from build123d import *

# Parameters (mm, degrees)
BASE_FLANGE1_DEPTH      = 25.4
BASE_FLANGE2_DEPTH      = 7.62
BASE_FLANGE2_DEPTH_BACK = 7.62
SKETCH9_R               = 2.159
CUT_EXTRUDE1_DEPTH      = 1.6764
SKETCH12_R              = 1.6764
SKETCH12_R_2            = 2.159
CUT_EXTRUDE4_DEPTH      = 1.6764
CUT_EXTRUDE5_DEPTH      = 2.54


# Sheet-metal steps are written as plain solids
with BuildPart() as part:
    # Sketch1 → Base-Flange1 (new body)
    with BuildSketch(Plane.XY):
        with BuildLine():
            Line((-52.705, -15.875), (-52.705, 15.3924))
            ThreePointArc((-52.705, 15.3924), (-52.563649733, 15.733649733), (-52.2224, 15.875))
            Line((-52.2224, 15.875), (52.2224, 15.875))
            ThreePointArc((52.2224, 15.875), (52.563649733, 15.733649733), (52.705, 15.3924))
            Line((52.705, 15.3924), (52.705, -15.875))
            Line((52.705, -15.875), (54.3814, -15.875))
            Line((54.3814, -15.875), (54.3814, 15.3924))
            ThreePointArc((54.3814, 15.3924), (53.749043541, 16.919043541), (52.2224, 17.5514))
            Line((52.2224, 17.5514), (-52.2224, 17.5514))
            ThreePointArc((-52.2224, 17.5514), (-53.749043541, 16.919043541), (-54.3814, 15.3924))
            Line((-54.3814, 15.3924), (-54.3814, -15.875))
            Line((-54.3814, -15.875), (-52.705, -15.875))
        make_face()
    extrude(amount=BASE_FLANGE1_DEPTH)


with BuildPart() as body_2:
    # Sketch6 → Base-Flange2 (new, two sides: drawn at the far end of the back side and taken through both)
    with BuildSketch(Plane(origin=(0, 0, 0), x_dir=(0, 0, -1), z_dir=(1, 0, 0)).offset(-BASE_FLANGE2_DEPTH_BACK)):
        with BuildLine():
            Line((-25.4, 15.875), (-68.0974, 15.875))
            ThreePointArc((-68.0974, 15.875), (-68.438649733, 15.733649733), (-68.58, 15.3924))
            Line((-68.58, 15.3924), (-68.58, 5.334))
            ThreePointArc((-68.58, 5.334), (-69.212356459, 3.807356459), (-70.739, 3.175))
            Line((-70.739, 3.175), (-99.06, 3.175))
            Line((-99.06, 3.175), (-99.06, 4.8514))
            Line((-99.06, 4.8514), (-70.739, 4.8514))
            ThreePointArc((-70.739, 4.8514), (-70.397750267, 4.992750267), (-70.2564, 5.334))
            Line((-70.2564, 5.334), (-70.2564, 15.3924))
            ThreePointArc((-70.2564, 15.3924), (-69.624043541, 16.919043541), (-68.0974, 17.5514))
            Line((-68.0974, 17.5514), (-25.4, 17.5514))
            Line((-25.4, 17.5514), (-25.4, 15.875))
        make_face()
    extrude(amount=BASE_FLANGE2_DEPTH + BASE_FLANGE2_DEPTH_BACK)

    # Sketch9 → Cut-Extrude1 (cut)
    with BuildSketch(Plane(origin=(0, 4.8514, 0), x_dir=(1, 0, 0), z_dir=(0, 1, 0))):
        with Locations(Location((0, -78.3844, 0), (0, 0, 270))):
            Circle(SKETCH9_R)
        with Locations(Location((0, -93.4466, 0), (0, 0, 270))):
            Circle(SKETCH9_R)
    extrude(amount=-CUT_EXTRUDE1_DEPTH, mode=Mode.SUBTRACT)


with BuildPart() as cut_extrude4_tool:
    # Sketch12 → Cut-Extrude4 (new body)
    with BuildSketch(Plane(origin=(0, 17.5514, 0), x_dir=(1, 0, 0), z_dir=(0, 1, 0))):
        with Locations(Location((0, -57.15, 0), (0, 0, 270))):
            Circle(SKETCH12_R)
        with Locations(Location((-41.49725, -12.7, 0), (0, 0, 270))):
            Circle(SKETCH12_R_2)
        with Locations(Location((41.49725, -12.7, 0), (0, 0, 270))):
            Circle(SKETCH12_R_2)
    extrude(amount=-CUT_EXTRUDE4_DEPTH)


with BuildPart() as part_1:
    add(part.part)

    # Cut-Extrude4: cut by cut_extrude4_tool
    add(cut_extrude4_tool.part, mode=Mode.SUBTRACT)


with BuildPart() as body_2_1:
    add(body_2.part)

    # Cut-Extrude4: cut by cut_extrude4_tool
    add(cut_extrude4_tool.part, mode=Mode.SUBTRACT)


with BuildPart() as cut_extrude5_tool:
    # Sketch12<3> → Cut-Extrude5 (new body)
    with BuildSketch(Plane(origin=(0, 17.5514, 0), x_dir=(1, 0, 0), z_dir=(0, 1, 0))):
        with BuildLine():
            Line((-1.6764, -25.4), (1.6764, -25.4))
            ThreePointArc((1.6764, -25.4), (0, -23.7236), (-1.6764, -25.4))
        make_face()
        with BuildLine():
            ThreePointArc((-1.6764, -25.4), (0, -27.0764), (1.6764, -25.4))
            Line((1.6764, -25.4), (-1.6764, -25.4))
        make_face()
    extrude(amount=-CUT_EXTRUDE5_DEPTH)


with BuildPart() as part_2:
    add(part_1.part)

    # Cut-Extrude5: cut by cut_extrude5_tool
    add(cut_extrude5_tool.part, mode=Mode.SUBTRACT)


with BuildPart() as body_2_2:
    add(body_2_1.part)

    # Cut-Extrude5: cut by cut_extrude5_tool
    add(cut_extrude5_tool.part, mode=Mode.SUBTRACT)

    # Combine1: union part
    add(part_2.part)


solid = body_2_2.part
Check sheet for the modelled part. Datum: model origin and axes. Units: mm. A direction names the side the tool comes from. Coordinates: 2 decimals unless noted, no trailing zeros. Write each loop counter-clockwise with the first axis right and the second up, starting at its lowest first coordinate (ties: lowest second). Pieces come first, ordered by that corner, then holes.
Item 1: Mould release check, pull along X, two halves, no side actions. Record for faces 1 (the face through (0, 3.175, 85)), 2 (the face through (7.62, 16.3, 62.1)), 3 (the face through (-52.705, 0, 13)), 4 (the face through (-42.811, 16.725, 10.987)): released by +X, released by -X, zero draft, split by the parting line, or undercut.
Numbers:
face 1: zero draft
face 2: released by +X
face 3: undercut
face 4: undercut
Item 2: Cross-section at D-D on y = -10. Record the boundary of the cut face in (x, z) (3 decimals).
Numbers:
outline: (-54.381, 0) - (-52.705, 0) - (-52.705, 25.4) - (-54.381, 25.4) - close; (52.705, 0) - (54.381, 0) - (54.381, 25.4) - (52.705, 25.4) - close
Item 3: Cross-section at A-A on y = 14. Record the boundary of the cut face in (x, z) (3 decimals).
Numbers:
outline: (-54.381, 0) - (-52.705, 0) - (-52.705, 25.4) - (-54.381, 25.4) - close; (-7.62, 68.58) - (7.62, 68.58) - (7.62, 70.256) - (-7.62, 70.256) - close; (52.705, 0) - (54.381, 0) - (54.381, 25.4) - (52.705, 25.4) - close
Item 4: Cross-section at C-C on x = 0. Record the boundary of the cut face in (y, z) (3 decimals), then the cut area to 3 significant figures.
Numbers:
outline: (3.175, 70.739) arc R2.159 ccw to (5.334, 68.58) - (15.392, 68.58) arc R0.483 cw to (15.875, 68.097) - (15.875, 58.826) - (17.551, 58.826) - (17.551, 68.097) arc R2.159 ccw to (15.392, 70.256) - (5.334, 70.256) arc R0.483 cw to (4.851, 70.739) - (4.851, 76.225) - (3.175, 76.225) - close; (3.175, 80.543) - (4.851, 80.543) - (4.851, 91.288) - (3.175, 91.288) - close; (3.175, 95.606) - (4.851, 95.606) - (4.851, 99.06) - (3.175, 99.06) - close; (15.875, 0) - (17.551, 0) - (17.551, 23.724) - (15.875, 23.724) - close; (15.875, 27.076) - (17.551, 27.076) - (17.551, 55.474) - (15.875, 55.474) - close
area: 160 mm2
Item 5: Access from +Z, -Z, +X, -X, +Y, -Y to the whole of each face (thin tool, end or side, straight path). Record for faces 5 (the face through (-1, 15.875, 18)), 6 (the face through (41, 17, 25.4)), 7 (the face through (-42, 17, 25.4)), 8 (the face through (0, 10, 70.256)).
Numbers:
face 5: -Z, -Y
face 6: +Z, +X, +Y, -Y
face 7: +Z, -X, +Y, -Y
face 8: +Z, +X, -X, +Y
Item 6: Scan lines: probe 1 along X at (y, z) = (12, 22.5) (3 decimals); probe 2 along X at (y, z) = (17.25, 57.15); probe 3 along Z at (x, y) = (46.5, 16.5). Record each from-to range of solid material in increasing order.
Numbers:
probe 1: x = -54.381 to -52.705, 52.705 to 54.381
probe 2: x = -7.62 to -1.68, 1.68 to 7.62
probe 3: z = 0 to 25.4
Item 7: Depth check by flat-ended pin: pin 1 Ø5.5 at (x, z) = (-41.5, 12.7) entering from +Y; pin 2 Ø10 at (x, y) = (-10.5, 2.5) entering from -Z; pin 3 Ø8 at (x, y) = (-3, 10.5) entering from +Z; pin 4 Ø17 at (x, z) = (3.5, 80) entering from +Y. Enter the tip coordinate at first touch or a pass-through.
Numbers:
pin 1: stops at y = 17.55
pin 2: stops at z = 68.58
pin 3: stops at z = 70.26
pin 4: stops at y = 4.85
Item 8: Cross-section at B-B on z = 57.15. Record the boundary of the cut face in (x, y) (3 decimals), then the cut area to 3 significant figures.
Numbers:
outline: (-7.62, 15.875) - (-1.676, 15.875) - (-1.676, 17.551) - (-7.62, 17.551) - close; (1.676, 15.875) - (7.62, 15.875) - (7.62, 17.551) - (1.676, 17.551) - close
area: 19.9 mm2
